CAD build for the part. Positions are in the model's coordinates, mm. Face numbers are marked on the shaded views. A direction names the side the tool comes from. Give positions to 0.01 mm unless a question says otherwise; leave off trailing zeros. Loops run counter-clockwise (first coordinate to the right, second up) from the corner with the lowest first, then second, coordinate; pieces in that order, holes last.
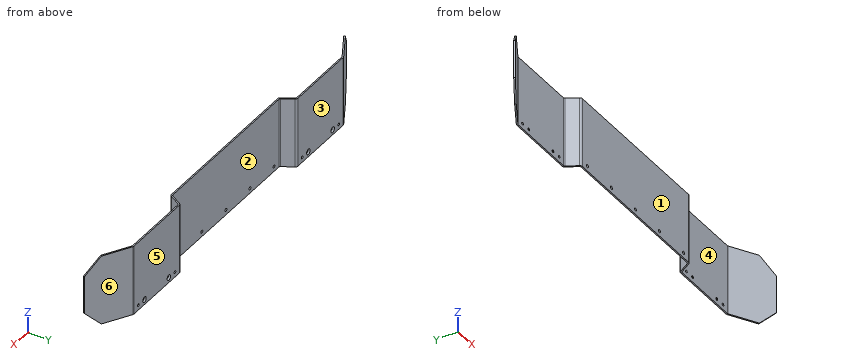
```python
from build123d import *

# Parameters (mm, degrees)
BASE_FLANGE1_DEPTH = 166.61684
SKETCH2_R          = 3.5
CUT_EXTRUDE1_DEPTH = 3.26
CHAMFER1_SIZE      = 38.1
SKETCH3_R          = 3
CUT_EXTRUDE2_DEPTH = 3.26
SKETCH8_R          = 3.125
CUT_EXTRUDE7_DEPTH = 10
CHAMFER2_SIZE      = 3.5


# Sheet-metal steps are written as plain solids
with BuildPart() as part:
    # Sketch1 → Base-Flange1 (new body)
    with BuildSketch(Plane.XY):
        with BuildLine():
            Line((-482.6, -24.572383929), (-388.340998066, 29.848076211))
            ThreePointArc((-388.340998066, 29.848076211), (-387.617455201, 30.147777479), (-386.840998066, 30.25))
            Line((-386.840998066, 30.25), (-219.196896451, 30.25))
            ThreePointArc((-219.196896451, 30.25), (-217.696896451, 29.848076211), (-216.598820239, 28.75))
            Line((-216.598820239, 28.75), (-201.807106343, 3.13))
            ThreePointArc((-201.807106343, 3.13), (-199.515787315, 0.838680972), (-196.385787315, 0))
            Line((-196.385787315, 0), (196.385787315, 0))
            ThreePointArc((196.385787315, 0), (199.515787315, 0.838680972), (201.807106343, 3.13))
            Line((201.807106343, 3.13), (216.598820239, 28.75))
            ThreePointArc((216.598820239, 28.75), (217.696896451, 29.848076211), (219.196896451, 30.25))
            Line((219.196896451, 30.25), (386.840998066, 30.25))
            ThreePointArc((386.840998066, 30.25), (387.617455201, 30.147777479), (388.340998066, 29.848076211))
            Line((388.340998066, 29.848076211), (482.6, -24.572383929))
            Line((482.6, -24.572383929), (484.23, -21.749141113))
            Line((484.23, -21.749141113), (389.970998066, 32.671319028))
            ThreePointArc((389.970998066, 32.671319028), (388.461205288, 33.296695673), (386.840998066, 33.51))
            Line((386.840998066, 33.51), (219.196896451, 33.51))
            ThreePointArc((219.196896451, 33.51), (216.066896451, 32.671319028), (213.775577423, 30.38))
            Line((213.775577423, 30.38), (198.983863526, 4.76))
            ThreePointArc((198.983863526, 4.76), (197.885787315, 3.661923789), (196.385787315, 3.26))
            Line((196.385787315, 3.26), (-196.385787315, 3.26))
            ThreePointArc((-196.385787315, 3.26), (-197.885787315, 3.661923789), (-198.983863526, 4.76))
            Line((-198.983863526, 4.76), (-213.775577423, 30.38))
            ThreePointArc((-213.775577423, 30.38), (-216.066896451, 32.671319028), (-219.196896451, 33.51))
            Line((-219.196896451, 33.51), (-386.840998066, 33.51))
            ThreePointArc((-386.840998066, 33.51), (-388.461205288, 33.296695673), (-389.970998066, 32.671319028))
            Line((-389.970998066, 32.671319028), (-484.23, -21.749141113))
            Line((-484.23, -21.749141113), (-482.6, -24.572383929))
        make_face()
    extrude(amount=BASE_FLANGE1_DEPTH)

    # Sketch2 → Cut-Extrude1 (cut)
    with BuildSketch(Plane(origin=(0, 3.26, 0), x_dir=(1, 0, 0), z_dir=(0, 1, 0))):
        with Locations(Location((0, -11.96, 0), (0, 0, 270))):
            Circle(SKETCH2_R)
        with Locations(Location((-177.8, -11.96, 0), (0, 0, 270))):
            Circle(SKETCH2_R)
        with Locations(Location((-88.9, -11.96, 0), (0, 0, 270))):
            Circle(SKETCH2_R)
        with Locations(Location((88.9, -11.96, 0), (0, 0, 270))):
            Circle(SKETCH2_R)
        with Locations(Location((177.8, -11.96, 0), (0, 0, 270))):
            Circle(SKETCH2_R)
    extrude(amount=-CUT_EXTRUDE1_DEPTH, mode=Mode.SUBTRACT)

    # Chamfer1
    chamfer1_edges = [part.edges().sort_by_distance(p)[0] for p in [
        (-483.415, -23.160762521, 166.61684),
        (-483.415, -23.160762521, 0),
        (483.415, -23.160762521, 0),
        (483.415, -23.160762521, 166.61684),
    ]]
    chamfer(chamfer1_edges, length=CHAMFER1_SIZE)

    # Sketch3 → Cut-Extrude2 (cut)
    with BuildSketch(Plane(origin=(0, 33.51, 0), x_dir=(1, 0, 0), z_dir=(0, 1, 0))):
        with Locations(Location((-258.045033443, -12.066000028, 0), (0, 0, 180))):
            Circle(SKETCH3_R)
        with Locations(Location((-348.045033443, -12.066000028, 0), (0, 0, 180))):
            Circle(SKETCH3_R)
        with Locations(Location((258.045033443, -12.066000028, 0), (0, 0, 180))):
            Circle(SKETCH3_R)
        with Locations(Location((348.045033443, -12.066000028, 0), (0, 0, 180))):
            Circle(SKETCH3_R)
    extrude(amount=-CUT_EXTRUDE2_DEPTH, mode=Mode.SUBTRACT)

    # Sketch8 → Cut-Extrude7 (cut)
    with BuildSketch(Plane(origin=(0, 33.51, 0), x_dir=(1, 0, 0), z_dir=(0, 1, 0))):
        with Locations(Location((235.448800169, -12.066000028, 0), (0, 0, 180))):
            Circle(SKETCH8_R)
        with Locations(Location((370.641266718, -12.066000028, 0), (0, 0, 180))):
            Circle(SKETCH8_R)
        with Locations(Location((-370.641266718, -12.066000028, 0), (0, 0, 180))):
            Circle(SKETCH8_R)
        with Locations(Location((-235.448800169, -12.066000028, 0), (0, 0, 180))):
            Circle(SKETCH8_R)
    extrude(amount=-CUT_EXTRUDE7_DEPTH, mode=Mode.SUBTRACT)

    # Chamfer2
    # the kernel refuses this chamfer: 3.5 mm, written as the material it takes off along each edge
    with BuildSketch(Plane(origin=(-348.045033443, 33.51, 12.066000028), x_dir=(-1, 0, 0), z_dir=(0, 0, -1))) as chamfer2_piece_1:
        Polygon((3 + CHAMFER2_SIZE, 0), (3, -CHAMFER2_SIZE), (3, 0), align=None)
    revolve(axis=Axis((-348.045033443, 33.51, 12.066000028), (0, 1, 0)), mode=Mode.SUBTRACT)
    with BuildSketch(Plane(origin=(-258.045033443, 33.51, 12.066000028), x_dir=(-1, 0, 0), z_dir=(0, 0, -1))) as chamfer2_piece_2:
        Polygon((3 + CHAMFER2_SIZE, 0), (3, -CHAMFER2_SIZE), (3, 0), align=None)
    revolve(axis=Axis((-258.045033443, 33.51, 12.066000028), (0, 1, 0)), mode=Mode.SUBTRACT)
    with BuildSketch(Plane(origin=(348.045033443, 33.51, 12.066000028), x_dir=(-1, 0, 0), z_dir=(0, 0, -1))) as chamfer2_piece_3:
        Polygon((3 + CHAMFER2_SIZE, 0), (3, -CHAMFER2_SIZE), (3, 0), align=None)
    revolve(axis=Axis((348.045033443, 33.51, 12.066000028), (0, 1, 0)), mode=Mode.SUBTRACT)
    with BuildSketch(Plane(origin=(258.045033443, 33.51, 12.066000028), x_dir=(-1, 0, 0), z_dir=(0, 0, -1))) as chamfer2_piece_4:
        Polygon((3 + CHAMFER2_SIZE, 0), (3, -CHAMFER2_SIZE), (3, 0), align=None)
    revolve(axis=Axis((258.045033443, 33.51, 12.066000028), (0, 1, 0)), mode=Mode.SUBTRACT)


solid = part.part
```
1. Saw through at D-D, the plane z = 150.5. List the corners of the cut face in (x, y), and give its area (3 significant figures).
Responses:
outline: (-465.19, -10.76) - (-463.56, -13.58) - (-388.34, 29.85) arc R3 cw to (-386.84, 30.25) - (-219.2, 30.25) arc R3 cw to (-216.6, 28.75) - (-201.81, 3.13) arc R6.26 ccw to (-196.39, 0) - (196.39, 0) arc R6.26 ccw to (201.81, 3.13) - (216.6, 28.75) arc R3 cw to (219.2, 30.25) - (386.84, 30.25) arc R3 cw to (388.34, 29.85) - (463.56, -13.58) - (465.19, -10.76) - (389.97, 32.67) arc R6.26 ccw to (386.84, 33.51) - (219.2, 33.51) arc R6.26 ccw to (213.78, 30.38) - (198.98, 4.76) arc R3 cw to (196.39, 3.26) - (-196.39, 3.26) arc R3 cw to (-198.98, 4.76) - (-213.78, 30.38) arc R6.26 ccw to (-219.2, 33.51) - (-386.84, 33.51) arc R6.26 ccw to (-389.97, 32.67) - close
area: 3,210 mm2
2. Pull direction X, two halves, no side cores. Call the marked faces 4, 5 and 6: released by +X, released by -X, zero draft, split by the parting line, or undercut.
Responses:
face 4: undercut
face 5: zero draft
face 6: released by +X
3. Drop flat-ended pins along their axis: pin 1 (4 mm diameter, centred on y = 14.5, z = 120.5, fed in from -X); pin 2 (9 mm diameter, centred on x = 177.8, z = 11.96, fed in from -Y); pin 3 (4 mm diameter, centred on x = 88.9, z = 11.96, fed in from -Y); pin 4 (1.5 mm diameter, centred on x = 128.5, z = 95.5, fed in from +Y). Give the stop position or say it passes through.
Responses:
pin 1: stops at x = -424.91
pin 2: stops at y = 0
pin 3: passes through
pin 4: stops at y = 3.26
4. Saw through at B-B, the plane z = 48.5. List the corners of the cut face in (x, y).
Responses:
outline: (-484.23, -21.75) - (-482.6, -24.57) - (-388.34, 29.85) arc R3 cw to (-386.84, 30.25) - (-219.2, 30.25) arc R3 cw to (-216.6, 28.75) - (-201.81, 3.13) arc R6.26 ccw to (-196.39, 0) - (196.39, 0) arc R6.26 ccw to (201.81, 3.13) - (216.6, 28.75) arc R3 cw to (219.2, 30.25) - (386.84, 30.25) arc R3 cw to (388.34, 29.85) - (482.6, -24.57) - (484.23, -21.75) - (389.97, 32.67) arc R6.26 ccw to (386.84, 33.51) - (219.2, 33.51) arc R6.26 ccw to (213.78, 30.38) - (198.98, 4.76) arc R3 cw to (196.39, 3.26) - (-196.39, 3.26) arc R3 cw to (-198.98, 4.76) - (-213.78, 30.38) arc R6.26 ccw to (-219.2, 33.51) - (-386.84, 33.51) arc R6.26 ccw to (-389.97, 32.67) - close
5. Tool access for the marked faces 1, 2 and 3: list every direction of +Z, -Z, +X, -X, +Y, -Y with a clear straight run to the whole face (end or side of a thin tool).
Responses:
face 1: +Z, -Z, -Y
face 2: +Z, -Z, +Y
face 3: +Z, -Z, +X, -X, +Y
6. Saw through at A-A, the plane y = 13. List the corners of the cut face in (x, z).
Responses:
outline: (-424.04, 0) - (-417.52, 0) - (-417.52, 166.62) - (-424.04, 166.62) - close; (-207.51, 0) - (-203.74, 0) - (-203.74, 166.62) - (-207.51, 166.62) - close; (203.74, 0) - (207.51, 0) - (207.51, 166.62) - (203.74, 166.62) - close; (417.52, 0) - (424.04, 0) - (424.04, 166.62) - (417.52, 166.62) - close
7. Probe line 1 along X through (y, z) = (20, 137); line 2 along X through (y, z) = (28, 56); line 3 along Z through (x, y) = (-177.8, 2.1). List the from-to ranges inside material, lowest first.
Responses:
line 1: x = -411.92 to -405.4, -211.55 to -207.78, 207.78 to 211.55, 405.4 to 411.92
line 2: x = -398.06 to -391.54, -216.17 to -212.4, 212.4 to 216.17, 391.54 to 398.06
line 3: z = 0 to 8.46, 15.46 to 166.62
8. Saw through at C-C, the plane x = -302. List the corners of the cut face in (y, z).
Responses:
outline: (30.25, 0) - (33.51, 0) - (33.51, 166.62) - (30.25, 166.62) - close
